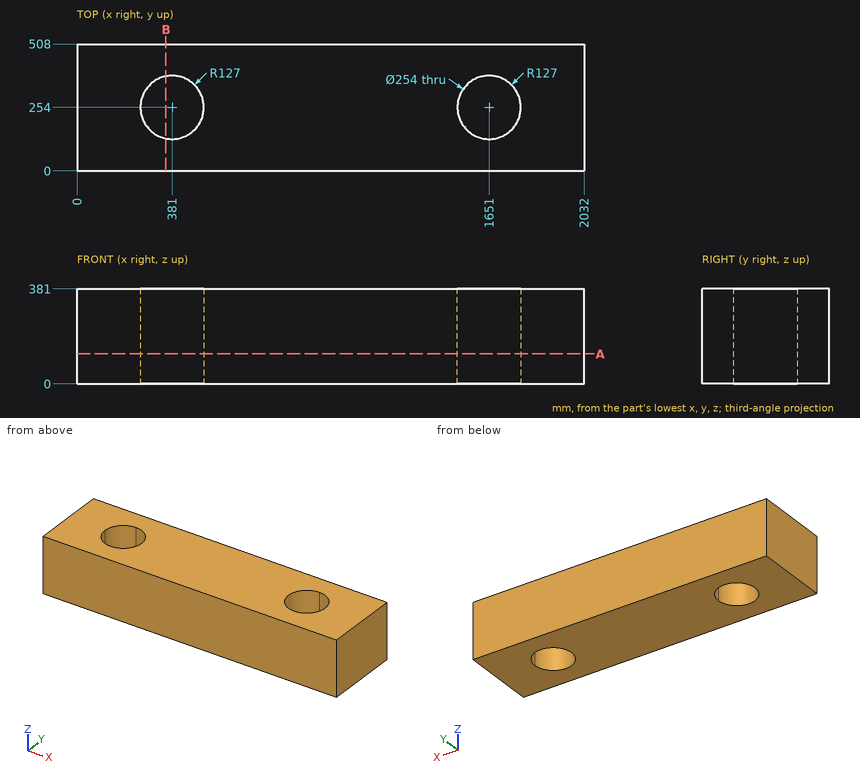
Here's the drawing with two shaded views (mm, measured from the low corner). I have some questions. Coordinates: 2 decimals unless noted, no trailing zeros. Order: outer loops, then holes, each group sorted by start corner. A loop starts at its lowest first (then second) coordinate and runs counter-clockwise, first axis right, second up. Notation, with made-up numbers: M -23,-6 L -10,-6 A17 ccw -10,20 Z; hole C 33,74.5 d5. An arc over 180 degrees is marked long. Write item = value, one per line.
(1) Suppose I cut it at B-B on x = 356. Please give me the cut outline in (y, z), plus the area to 3 significant figures.
Results are:
outline = M 0,0 L 129.48,0 L 129.48,381 L 0,381 Z; M 378.52,0 L 508,0 L 508,381 L 378.52,381 Z
area = 98,700 mm2
(2) Suppose I cut it at A-A on z = 120. Please give me the cut outline in (x, y), plus the area to 3 significant figures.
Results are:
outline = M 0,0 L 2032,0 L 2032,508 L 0,508 Z; hole M 254,254 A127 ccw long 381,381 A127 ccw Z; hole C 1651,254 d254
area = 931,000 mm2
(3) I need wall thicknesses on line 1 along X through (y, z) = (252, 141.5); line 2 along Y through (x, z) = (1651, 146.5); line 3 along X through (y, z) = (190, 280). Which ranges of each line are inside material? Lowest first, please. Write a range as [from, to].
Results are:
line_1 = [0, 254.02], [507.98, 1524.02], [1777.98, 2032]
line_2 = [0, 127], [381, 508]
line_3 = [0, 271.3], [490.7, 1541.3], [1760.7, 2032]
(4) For pin 1 Ø5 at (y, z) = (165.5, 247.5) entering from -X, with a flat end and sliding along its axis, tell me the tip position at first contact or that it passes through.
Results are:
pin_1 = 0
